from build123d import *

# Parameters (mm, degrees)
SKETCH1_R           = 0.875
BOSS_EXTRUDE1_DEPTH = 4
CUT_EXTRUDE1_DEPTH  = 10


with BuildPart() as part:
    # Sketch1 → Boss-Extrude1 (new body)
    with BuildSketch(Plane.XY):
        with BuildLine():
            Line((-27.646606378, 17.766968108), (-1.871361719, 12.611919177))
            ThreePointArc((-1.871361719, 12.611919177), (-12.502403615, 2.500480723), (-6.578148963, -10.92201704))
            Line((-6.578148963, -10.92201704), (-32.353393622, -5.766968108))
            ThreePointArc((-32.353393622, -5.766968108), (-41.766968108, 8.353393622), (-27.646606378, 17.766968108))
        make_face()
        with Locations((-40.296097095, 8.059219419)):
            Circle(SKETCH1_R, mode=Mode.SUBTRACT)
        with Locations((-18.625264162, 14.432993811)):
            Circle(SKETCH1_R, mode=Mode.SUBTRACT)
        with Locations((-22.743703, -6.159200379)):
            Circle(SKETCH1_R, mode=Mode.SUBTRACT)
    extrude(amount=BOSS_EXTRUDE1_DEPTH)

    # Sketch2 → Cut-Extrude1 (cut)
    with BuildSketch(Plane(origin=(0, 0, 0), x_dir=(-1, 0, 0), z_dir=(0, 0, -1))):
        Polygon((7.192307692, -9.461538462), (7.961538462, -11.307692308), (6.115384615, -12.076923077), (5.346153846, -10.230769231), align=None)
    extrude(amount=-CUT_EXTRUDE1_DEPTH, mode=Mode.SUBTRACT)


solid = part.part
For this review, take the finished solid that the model builds, in its own axes (mm). Round coordinates to 2 decimals unless told otherwise and drop trailing zeros. Write each loop counter-clockwise with the first axis right and the second up, starting at its lowest first coordinate (ties: lowest second). Pieces come first, ordered by that corner, then holes. Notation, with made-up numbers: (-31.75, 49) - (-12.75, 49) arc R25 ccw to (-12.75, 70) - close; hole circle Ø7 at (13.25, -8). An arc over 180 degrees is marked (long way). Use a Markdown table: item, result.
Q1. We need section C-C (x = -30). Give the boundary of the cut face in (y, z).
Derived:
| item | result |
|---|---|
| outline | (-6.24, 0) - (18, 0) - (18, 4) - (-6.24, 4) - close |
Q2. The part is to be moulded in two halves that separate along X. For faces 1 (the flat face through (-19.858, -8.266, 1.972)), 2 (the cylindrical face through (-18.222, 13.657, 1.972)), 3 (the flat face through (-14.939, 15.226, 1.972)), say which applies: pulls with the +X half, pulls with the -X half, needs draft (parallel to the pull), parting line crosses it, or undercut.
Derived:
| item | result |
|---|---|
| face 1 | pulls with the -X half |
| face 2 | undercut |
| face 3 | pulls with the +X half |
Q3. We need section A-A (z = 1.3). Give the boundary of the cut face in (x, y) (3 decimals), plus the area to 3 significant figures.
Derived:
| item | result |
|---|---|
| outline | (-32.353, -5.767) - (-7.707, -10.696) - (-7.535, -10.285) arc R12.75 cw to (-1.871, 12.612) - (-27.647, 17.767) arc R12 ccw to start; hole circle Ø1.75 at (-40.296, 8.059); hole circle Ø1.75 at (-22.744, -6.159); hole circle Ø1.75 at (-18.625, 14.433) |
| area | 702 mm2 |
Q4. Wall thickness on line 1 along Y through (x, z) = (-9.5, 0.5); line 2 along Y through (x, z) = (-9, 2.2); line 3 along X through (y, z) = (8, 1.55): over which ranges is each line inside the solid? List them lowest first.
Derived:
| item | result |
|---|---|
| line 1 | y = -10.34 to -8.5, 8.5 to 14.14 |
| line 2 | y = -10.44 to -9.03, 9.03 to 14.04 |
| line 3 | x = -41.83 to -41.17, -39.42 to -9.93 |
Q5. We need section B-B (y = 6). Give the boundary of the cut face in (x, z), plus the area to 3 significant figures.
Derived:
| item | result |
|---|---|
| outline | (-42, 0) - (-11.25, 0) - (-11.25, 4) - (-42, 4) - close |
| area | 123 mm2 |
Q6. Clearance check with flat-ended pins moving along their axes: pin 1 (1.5 mm diameter, centred on x = -37, z = 2, fed in from -Y); pin 2 (2 mm diameter, centred on x = -21, z = 2.5, fed in from -Y). State where each tip first meets the part, or that it passes through.
Derived:
| item | result |
|---|---|
| pin 1 | stops at y = -4.24 |
| pin 2 | stops at y = -8.24 |
